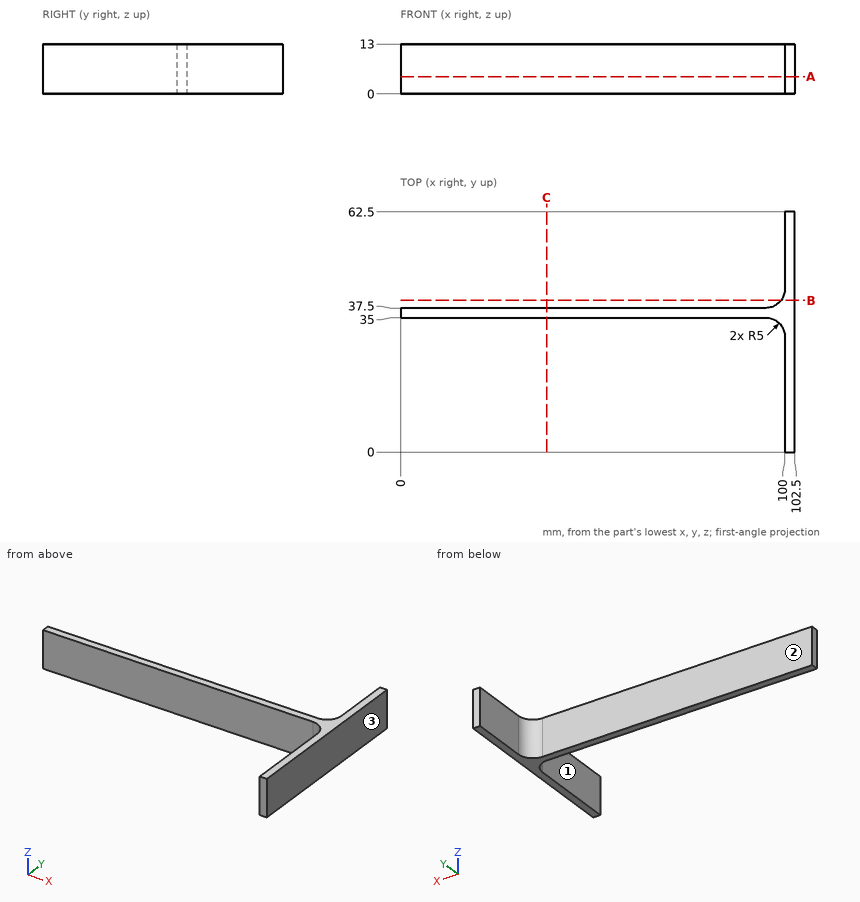
Check sheet for the drawn part. Datum: minimum x, y, z corner. Units: mm. A direction names the side the tool comes from. Coordinates: 2 decimals unless noted, no trailing zeros. Write each loop counter-clockwise with the first axis right and the second up, starting at its lowest first coordinate (ties: lowest second). Pieces come first, ordered by that corner, then holes. Notation, with made-up numbers: M 75,14 L 132,14 A13 cw 132,37 Z; hole C 63,-9.75 d9. An arc over 180 degrees is marked long. One line per item, written item: value.
Item 1: Section check B-B, the plane y = 39.5. Record the boundary of the cut face in (x, z).
Check sheet entries:
outline: M 99,0 L 102.5,0 L 102.5,13 L 99,13 Z
Item 2: Scan lines: line 1 along X through (y, z) = (29, 9.5); line 2 along Y through (x, z) = (74, 12.25). Record each from-to range of solid material in increasing order.
Check sheet entries:
line 1: x = 100 to 102.5
line 2: y = 35 to 37.5
Item 3: Section check A-A, the plane z = 4.5. Record the boundary of the cut face in (x, y), plus the area to 3 significant figures.
Check sheet entries:
outline: M 0,35 L 95,35 A5 cw 100,30 L 100,0 L 102.5,0 L 102.5,62.5 L 100,62.5 L 100,42.5 A5 cw 95,37.5 L 0,37.5 Z
area: 417 mm^2
Item 4: Access from +Z, -Z, +X, -X, +Y, -Y to the whole of each face (thin tool, end or side, straight path). Record for the marked faces 1, 2 and 3.
Check sheet entries:
face 1: +Z, -Z, -X, -Y
face 2: +Z, -Z, -X, +Y
face 3: +Z, -Z, +X, +Y, -Y
Item 5: Gauge pin test, flat ends, axial feed: pin 1 Ø12 at (x, y) = (23.5, 45.5) entering from -Z; pin 2 Ø6.5 at (x, z) = (48.5, 9.5) entering from +Y. Record the tip position at first contact, or that the pin passes through.
Check sheet entries:
pin 1: passes through
pin 2: stops at y = 37.5
Item 6: Section check C-C, the plane x = 38. Record the boundary of the cut face in (y, z).
Check sheet entries:
outline: M 35,0 L 37.5,0 L 37.5,13 L 35,13 Z
